Source: CAD feature listing. Evaluate the final solid. Frame: model axes, mm. Round coordinates to 2 decimals unless told otherwise and drop trailing zeros. Order: outer loops, then holes, each group sorted by start corner. A loop starts at its lowest first (then second) coordinate and runs counter-clockwise, first axis right, second up. Notation, with made-up numbers: (24, -26) -> (64, -26) arc R16 cw to (64, -13) -> close; hole circle Ø2 at (44.5, 4.5). An arc over 180 degrees is marked (long way). One line per item, written item: value. Start each with the question number.
1) Section C-C (x = 9). Return the cut outline in (y, z) (3 decimals), and give its area (3 significant figures).
2) Mould query, pull axis Y, two halves, no side actions, for faces 1 (the face through (2.06, 24.5, 3.22)), 2 (the face through (38, 50.8, 3)), 3 (the face through (73.81, 24.78, 3.22)), 4 (the face through (38, 26, 7.62)). Classes: pulls with the +Y half, pulls with the -Y half, needs draft (parallel to the pull), parting line crosses it, or undercut.
3) Pin query (flat end, axial travel): P1, Ø1, axis at x = 39, z = 7, coming from the -Y side (3 decimals); P2, Ø3, axis at x = 61, z = 6.5, coming from the +Y side; P3, Ø0.6, axis at x = 28, z = 7, coming from the +Y side (3 decimals); P4, Ø2.5, axis at x = 38.1, y = 49.21, coming from the +Z side. Return the tip coordinate at first contact, or that it passes through.
4) Ray query, L1, parallel to Y at x = 38.1, z = 1.5; L2, parallel to X at y = 26, z = 1; L3, parallel to X at y = 24.5, z = 6.25. Return the intervals inside material, ascending.
5) Section A-A (y = 25.4). State how many separate pieces and enclosed holes the cut face has, and give its area (3 significant figures).
```python
from build123d import *

# Parameters (mm, degrees)
SKETCH1_W           = 76.2
SKETCH1_H           = 50.8
BOSS_EXTRUDE1_DEPTH = 7.62
CUT_EXTRUDE3_DEPTH  = 1.27
SKETCH5_R           = 1.016
CUT_EXTRUDE4_DEPTH  = 92.800885072


with BuildPart() as part:
    # Sketch1 → Boss-Extrude1 (new body)
    with BuildSketch(Plane.XY):
        with Locations((38.1, 25.4)):
            Rectangle(SKETCH1_W, SKETCH1_H)
    extrude(amount=BOSS_EXTRUDE1_DEPTH)

    # Sketch4 → Cut-Extrude3 (cut)
    with BuildSketch(Plane.XY.offset(7.62)):
        Polygon((38.1, 47.625), (38.1, 50.8), (0, 50.8), (0, 0), (38.1, 0), (38.1, 3.175), (3.175, 3.175), (3.175, 47.625), align=None)
        Polygon((76.2, 50.8), (38.1, 50.8), (38.1, 47.625), (73.025, 47.625), (73.025, 3.175), (38.1, 3.175), (38.1, 0), (76.2, 0), align=None)
    extrude(amount=-CUT_EXTRUDE3_DEPTH, mode=Mode.SUBTRACT)

    # Sketch5 → Cut-Extrude4 (cut, through all)
    with BuildSketch(Plane.XY.offset(6.35)):
        with Locations((1.5875, 25.4)):
            Circle(SKETCH5_R)
        with Locations((38.1, 49.2125)):
            Circle(SKETCH5_R)
        with Locations((74.6125, 25.4)):
            Circle(SKETCH5_R)
        with Locations((38.1, 1.5875)):
            Circle(SKETCH5_R)
    extrude(amount=-CUT_EXTRUDE4_DEPTH, mode=Mode.SUBTRACT)


solid = part.part
```
Findings:
1. outline: (0, 0) -> (50.8, 0) -> (50.8, 6.35) -> (47.625, 6.35) -> (47.625, 7.62) -> (3.175, 7.62) -> (3.175, 6.35) -> (0, 6.35) -> close
1. area: 379 mm2
2. face 1: undercut
2. face 2: pulls with the +Y half
2. face 3: undercut
2. face 4: needs draft
3. P1: y = 3.175
3. P2: y = 50.8
3. P3: y = 47.625
3. P4: z = 6.35
4. L1: 0 to 0.57, 2.6 to 48.2, 50.23 to 50.8
4. L2: 0 to 0.77, 2.41 to 73.79, 75.43 to 76.2
4. L3: 0 to 1.12, 2.06 to 74.14, 75.08 to 76.2
5. separate pieces: 3
5. enclosed holes: 0
5. area: 547 mm2
